```python
from build123d import *

# Parameters (mm, degrees)
BOSS_EXTRUDE1_DEPTH        = 20
BOSS_EXTRUDE2_DEPTH        = 20
FILLET1_R                  = 20
FILLET2_R                  = 25
FILLET3_R                  = 12
F_20_0_20_DIAMETER_HOLE1_D = 20
F_18_0_18_DIAMETER_HOLE1_D = 18


with BuildPart() as part:
    # Sketch1 → Boss-Extrude1 (new body)
    with BuildSketch(Plane(origin=(0, 0, 0), x_dir=(1, 0, 0), z_dir=(0, 1, 0))):
        Polygon((0, 0), (150, 0), (150, -75), (0, -35), align=None)
    extrude(amount=BOSS_EXTRUDE1_DEPTH)

    # Sketch2 → Boss-Extrude2 (add)
    with BuildSketch(Plane(origin=(0, 0, 0), x_dir=(-1, 0, 0), z_dir=(0, 0, -1))):
        Polygon((-50, 0), (-150, 0), (-150, 60), (-50, 80), align=None)
    extrude(amount=-BOSS_EXTRUDE2_DEPTH)

    # Fillet1
    fillet1_edges = [part.edges().sort_by_distance(p)[0] for p in [
        (0, 10, 35),
    ]]
    fillet(fillet1_edges, radius=FILLET1_R)

    # Fillet2
    fillet2_edges = [part.edges().sort_by_distance(p)[0] for p in [
        (50, 80, 10),
        (150, 10, 75),
    ]]
    fillet(fillet2_edges, radius=FILLET2_R)

    # Fillet3
    fillet3_edges = [part.edges().sort_by_distance(p)[0] for p in [
        (150, 60, 10),
    ]]
    fillet(fillet3_edges, radius=FILLET3_R)

    # Ø20.0 (20) Diameter Hole1 (through all)
    with Locations(Plane(origin=(0, 20, 0), x_dir=(1, 0, 0), z_dir=(0, 1, 0))):
        with Locations((20, -19.634433738), (125, -42.45970884)):
            Hole(F_20_0_20_DIAMETER_HOLE1_D / 2)

    # Ø18.0 (18) Diameter Hole1 (through all)
    with Locations(Plane.XY.offset(20)):
        with Locations((75, 49.504902432)):
            Hole(F_18_0_18_DIAMETER_HOLE1_D / 2)


solid = part.part
```
Source: CAD feature listing. Evaluate the final solid. Frame: model axes, mm. A direction names the side the tool comes from. Round coordinates to 2 decimals unless told otherwise and drop trailing zeros. Loops run counter-clockwise (first coordinate to the right, second up) from the corner with the lowest first, then second, coordinate; pieces in that order, holes last. Notation, with made-up numbers: M 59.5,85.25 L 114.5,85.25 A25 cw 114.5,97.25 Z; hole C 40.25,12 d10. An arc over 180 degrees is marked long. Use a Markdown table: item, result. Add a question column.
1. Cut plane D-D, the plane x = 125. Output: boundary loops of the cut face in (y, z).
2. Set-up query: faces 4 (the cylindrical face through (147.353, 57.681, 10.14)), 5 (the flat face through (50, 35, 10)), 6 (the flat face through (99, 42, 20)). Return all of +Z, -Z, +X, -X, +Y, -Y with unobstructed straight access to the full face (end or side cutting, diameter ignored); none if empty.
3. Pull-direction query (Z, two-part tool) for faces 1 (the cylindrical face through (132.94, 9.86, 48.54)), 2 (the flat face through (91, 28, 0)), 3 (the flat face through (150, 19, 16)); classes: +Z half, -Z half, draft (parallel to the pull), parting line (faces both ways), or undercut.
4. Cut plane B-B, the plane z = 24.5. Output: boundary loops of the cut face in (x, y).
5. Cut plane A-A, the plane x = 75. Output: boundary loops of the cut face in (y, z).
6. Cut plane C-C, the plane y = 13. Output: boundary loops of the cut face in (x, z), and give its area (3 significant figures).
7. Ray query, line 1 along Z through (x, y) = (125, 14.25); line 2 along Y through (x, z) = (75, 16); line 3 along Y through (x, z) = (93.5, 56.5). Return the intervals inside material, ascending. Write a range as [from, to].
8. Contact query for flat-ended pins moving along their axis: pin 1 (10 mm diameter, centred on x = 112.5, z = 24, fed in from +Y); pin 2 (10 mm diameter, centred on y = 27.5, z = 8, fed in from -X); pin 3 (16 mm diameter, centred on x = 75, y = 49.5, fed in from -Z); pin 4 (4 mm diameter, centred on y = 12, z = 51, fed in from +X). Output: stop coordinate, or through.
Solution:
| question | item | result |
|---|---|---|
| 1 | outline | M 0,0 L 65,0 L 65,20 L 20,20 L 20,32.46 L 0,32.46 Z; M 0,52.46 L 20,52.46 L 20,67.46 L 0,67.46 Z |
| 2 | face 4 | +Z, -Z, +X, +Y |
| 2 | face 5 | +Z, -Z, -X, +Y |
| 2 | face 6 | +Z, +X, -X, +Y |
| 3 | face 1 | undercut |
| 3 | face 2 | -Z half |
| 3 | face 3 | draft |
| 4 | outline | M 0.6,0 L 11.26,0 L 11.26,20 L 0.6,20 Z; M 28.74,0 L 150,0 L 150,20 L 28.74,20 Z |
| 5 | outline | M 0,0 L 40.5,0 L 40.5,20 L 20,20 L 20,55 L 0,55 Z; M 58.5,0 L 74.5,0 L 74.5,20 L 58.5,20 Z |
| 6 | outline | M 0,0 L 150,0 L 150,42.46 A25 ccw 118.56,66.62 L 14.85,38.96 A20 ccw 0,19.63 Z; hole C 20,19.63 d20; hole C 125,42.46 d20 |
| 6 | area | 7,340 mm2 |
| 7 | line 1 | z = [0, 32.46], [52.46, 67.46] |
| 7 | line 2 | y = [0, 40.5], [58.5, 74.5] |
| 7 | line 3 | y = [0, 20] |
| 8 | pin 1 | stops at y = 68.1 |
| 8 | pin 2 | stops at x = 50 |
| 8 | pin 3 | passes through |
| 8 | pin 4 | stops at x = 149.13 |
